Can you work these out from the model? Positions are in its coordinate system, mm. Coordinates: 2 decimals unless noted, no trailing zeros. Order: outer loops, then holes, each group sorted by start corner. A loop starts at its lowest first (then second) coordinate and runs counter-clockwise, first axis right, second up. Notation, with made-up numbers: (-12, 16) - (45, 16) arc R18 ccw to (45, 33) - close; hole circle Ø11 at (89.5, 76.5). An arc over 180 degrees is marked (long way). Use a Markdown table: item, result. Add a question column.
(1) I want a section at C-C (y = 1.5). List the corners of the cut face in (x, z) for me.
(2) If I drill on L1, parallel to Y at x = -10, z = 2.25; L2, parallel to X at y = -28, z = 0.55; L3, parallel to X at y = 10.5, z = 1.4, over which ranges is the centre line in solid material (lowest first)? Write a range as [from, to].
(3) For pin 1 Ø2 at (x, y) = (-76, 20.5) entering from -Z; pin 2 Ø3 at (x, y) = (110, 73) entering from +Z, each with a flat end and sliding along its axis, tell me the tip position at first contact or that it passes through.
(4) I want a section at D-D (x = -82). List the corners of the cut face in (y, z) for me, and give its area (3 significant figures).
(5) I want a section at A-A (y = 67). List the corners of the cut face in (x, z) for me, and give its area (3 significant figures).
(6) I want a section at B-B (x = -41). List the corners of the cut face in (y, z) for me.
```python
from build123d import *

# Parameters (mm, degrees)
MODEL_R             = 2
MODEL_W             = 130
MODEL_H             = 10
MODEL_W_2           = 15
MODEL_H_2           = 90
MODEL_W_3           = 25
MODEL_H_3           = 25
MODEL_H_4           = 30
MODEL_W_4           = 170
MODEL_H_5           = 4
EXTRUDE_1_DEPTH     = 3
SKETCH_1_R          = 2
CUT_EXTRUDE_1_DEPTH = 10


with BuildPart() as part:
    # Model → 凸台-拉伸1 (new body)
    with BuildSketch(Plane.XY):
        with BuildLine():
            Line((130, -77), (130, 77))
            ThreePointArc((130, 77), (129.121320344, 79.121320344), (127, 80))
            Line((127, 80), (-127, 80))
            ThreePointArc((-127, 80), (-129.121320344, 79.121320344), (-130, 77))
            Line((-130, 77), (-130, -77))
            ThreePointArc((-130, -77), (-129.121320344, -79.121320344), (-127, -80))
            Line((-127, -80), (127, -80))
            ThreePointArc((127, -80), (129.121320344, -79.121320344), (130, -77))
        make_face()
        with Locations((-110, 73)):
            Circle(MODEL_R, mode=Mode.SUBTRACT)
        with Locations((110, 73)):
            Circle(MODEL_R, mode=Mode.SUBTRACT)
        with Locations((110, -73)):
            Circle(MODEL_R, mode=Mode.SUBTRACT)
        with Locations((-110, -73)):
            Circle(MODEL_R, mode=Mode.SUBTRACT)
        with Locations((-120, 73)):
            Circle(MODEL_R, mode=Mode.SUBTRACT)
        with Locations((120, 73)):
            Circle(MODEL_R, mode=Mode.SUBTRACT)
        with Locations((-120, -73)):
            Circle(MODEL_R, mode=Mode.SUBTRACT)
        with Locations((120, -73)):
            Circle(MODEL_R, mode=Mode.SUBTRACT)
        with Locations((-100, 73)):
            Circle(MODEL_R, mode=Mode.SUBTRACT)
        with Locations((100, 73)):
            Circle(MODEL_R, mode=Mode.SUBTRACT)
        with Locations((-100, -73)):
            Circle(MODEL_R, mode=Mode.SUBTRACT)
        with Locations((100, -73)):
            Circle(MODEL_R, mode=Mode.SUBTRACT)
        with Locations((0, 65)):
            Rectangle(MODEL_W, MODEL_H, mode=Mode.SUBTRACT)
        with Locations((0, -65)):
            Rectangle(MODEL_W, MODEL_H, mode=Mode.SUBTRACT)
        with Locations((-110, 0)):
            Rectangle(MODEL_W_2, MODEL_H_2, mode=Mode.SUBTRACT)
        with Locations((65, 0)):
            Rectangle(MODEL_W_3, MODEL_H_3, mode=Mode.SUBTRACT)
        with Locations((-65, 0)):
            Rectangle(MODEL_W_3, MODEL_H_3, mode=Mode.SUBTRACT)
        with Locations((114.5, 0)):
            Rectangle(MODEL_W_2, MODEL_H_4, mode=Mode.SUBTRACT)
        with Locations((0, 29)):
            Rectangle(MODEL_W_4, MODEL_H_5, mode=Mode.SUBTRACT)
        with Locations((0, -29)):
            Rectangle(MODEL_W_4, MODEL_H_5, mode=Mode.SUBTRACT)
    extrude(amount=EXTRUDE_1_DEPTH)

    # 草图1 → 切除-拉伸1 (cut)
    with BuildSketch(Plane.XY.offset(3)):
        with Locations((-28.75, 43)):
            Circle(SKETCH_1_R)
        with Locations((28.75, 43)):
            Circle(SKETCH_1_R)
        with Locations((-28.75, -43)):
            Circle(SKETCH_1_R)
        with Locations((28.75, -43)):
            Circle(SKETCH_1_R)
    extrude(amount=-CUT_EXTRUDE_1_DEPTH, mode=Mode.SUBTRACT)


solid = part.part
```
Answers follow:
| question | item | result |
|---|---|---|
| 1 | outline | (-130, 0) - (-117.5, 0) - (-117.5, 3) - (-130, 3) - close; (-102.5, 0) - (-77.5, 0) - (-77.5, 3) - (-102.5, 3) - close; (-52.5, 0) - (52.5, 0) - (52.5, 3) - (-52.5, 3) - close; (77.5, 0) - (107, 0) - (107, 3) - (77.5, 3) - close; (122, 0) - (130, 0) - (130, 3) - (122, 3) - close |
| 2 | L1 | y = [-80, -70], [-60, -31], [-27, 27], [31, 60], [70, 80] |
| 2 | L2 | x = [-130, -117.5], [-102.5, -85], [85, 130] |
| 2 | L3 | x = [-130, -117.5], [-102.5, -77.5], [-52.5, 52.5], [77.5, 107], [122, 130] |
| 3 | pin 1 | stops at z = 0 |
| 3 | pin 2 | passes through |
| 4 | outline | (-80, 0) - (-31, 0) - (-31, 3) - (-80, 3) - close; (-27, 0) - (27, 0) - (27, 3) - (-27, 3) - close; (31, 0) - (80, 0) - (80, 3) - (31, 3) - close |
| 4 | area | 456 mm² |
| 5 | outline | (-130, 0) - (-65, 0) - (-65, 3) - (-130, 3) - close; (65, 0) - (130, 0) - (130, 3) - (65, 3) - close |
| 5 | area | 390 mm² |
| 6 | outline | (-80, 0) - (-70, 0) - (-70, 3) - (-80, 3) - close; (-60, 0) - (-31, 0) - (-31, 3) - (-60, 3) - close; (-27, 0) - (27, 0) - (27, 3) - (-27, 3) - close; (31, 0) - (60, 0) - (60, 3) - (31, 3) - close; (70, 0) - (80, 0) - (80, 3) - (70, 3) - close |
